Could you check a few things on this model? Use its own coordinates, in mm. A direction names the side the tool comes from. Coordinates: 2 decimals unless noted, no trailing zeros. Write each loop counter-clockwise with the first axis right and the second up, starting at its lowest first coordinate (ties: lowest second). Pieces come first, ordered by that corner, then holes. Notation, with made-up numbers: M 63.5,40 L 84.5,40 A30 cw 84.5,70 Z; hole C 48.25,49.5 d5. An arc over 180 degrees is marked long. Write item = value, one per line.
```python
from build123d import *

# Parameters (mm, degrees)
F1_DEPTH = 45
F2_T     = -2.5
F3_R     = 18
F4_DEPTH = 25
F5_R     = 20
F5_R_2   = 18
F6_DEPTH = 6


with BuildPart() as f1:
    # F0 (on Front) → F1 (new body)
    with BuildSketch(Plane.XZ):
        with BuildLine():
            Line((-26.5, -37.5), (26.5, -37.5))
            Line((26.5, -37.5), (26.5, 22.5))
            ThreePointArc((26.5, 22.5), (22.106602, 33.106602), (11.5, 37.5))
            Line((11.5, 37.5), (-11.5, 37.5))
            ThreePointArc((-11.5, 37.5), (-22.106602, 33.106602), (-26.5, 22.5))
            Line((-26.5, 22.5), (-26.5, -37.5))
        make_face()
    extrude(amount=F1_DEPTH)

    # F2
    f2_openings = [f1.faces().sort_by_distance(p)[0] for p in [
        (0, -45, -0.850304),
    ]]
    offset(amount=F2_T, openings=f2_openings)

    # F3 (on face) → F4 (cut)
    with BuildSketch(Plane(origin=(0, 0, 0), x_dir=(-1, 0, 0), z_dir=(0, 1, 0))):
        with Locations((0, 13)):
            Circle(F3_R)
    extrude(amount=-F4_DEPTH, mode=Mode.SUBTRACT)

    # F5 (on face) → F6 (join)
    with BuildSketch(Plane(origin=(0, 0, 0), x_dir=(-1, 0, 0), z_dir=(0, 1, 0))):
        with Locations((0, 13)):
            Circle(F5_R)
        with Locations((0, 13)):
            Circle(F5_R_2, mode=Mode.SUBTRACT)
    extrude(amount=F6_DEPTH)


solid = f1.part
```
Item 1: For faces 1 (the face through (-26.5, -22, -7)), 2 (the face through (-20.241, -23.452, 31.435)), which set-ups out of +Z, -Z, +X, -X, +Y, -Y let a thin tool reach every point of the face, with its end or its side?
Numbers:
face_1 = +Z, -Z, -X, +Y, -Y
face_2 = -Y
Item 2: Imagine slicing it at B-B (z = 13). Write out the boundary of the cut face in (x, y), and give its area (3 significant figures).
Numbers:
outline = M -26.5,-45 L -24,-45 L -24,-2.5 L -18,-2.5 L -18,6 L -20,6 L -20,0 L -26.5,0 Z; M 18,-2.5 L 24,-2.5 L 24,-45 L 26.5,-45 L 26.5,0 L 20,0 L 20,6 L 18,6 Z
area = 279 mm²
Item 3: If we mould it in two halves opening along Z, with no side actions, what happens to faces 3 (the face through (22.22, -22.18, 32.99)), 4 (the face through (-9.229, 2.958, -4.743)), 5 (the face through (-24, -23, -6))? For each: pulls with the +Z half, pulls with the -Z half, needs draft (parallel to the pull), parting line crosses it, or undercut.
Numbers:
face_3 = pulls with the +Z half
face_4 = parting line crosses it
face_5 = undercut
Item 4: Imagine slicing it at C-C (y = -24.5). Write out the boundary of the cut face in (x, z), and give its area (3 significant figures).
Numbers:
outline = M -26.5,-37.5 L 26.5,-37.5 L 26.5,22.5 A15 ccw 11.5,37.5 L -11.5,37.5 A15 ccw -26.5,22.5 Z; hole M -24,-35 L 24,-35 L 24,22.5 A12.5 ccw 11.5,35 L -11.5,35 A12.5 ccw -24,22.5 Z
area = 585 mm²
Item 5: I'm going to push flat-ended pins straight in: P1, Ø2, axis at x = 4, z = -26.5, coming from the -Y side; P2, Ø3, axis at x = 11.5, z = -10, coming from the +Y side. Where does each tip first touch, or does it pass through?
Numbers:
P1 = -2.5
P2 = 0
Item 6: Imagine slicing it at A-A (x = 0). Write out the boundary of the cut face in (y, z).
Numbers:
outline = M -45,-37.5 L 0,-37.5 L 0,-7 L 6,-7 L 6,-5 L -2.5,-5 L -2.5,-35 L -45,-35 Z; M -45,35 L -2.5,35 L -2.5,31 L 6,31 L 6,33 L 0,33 L 0,37.5 L -45,37.5 Z
Item 7: If I drill on line 1 along Z through (x, y) = (-10, -23.5); line 2 along X through (y, z) = (-32.5, -20); line 3 along Z through (x, y) = (0, -1), over which ranges is the centre line in solid material (lowest first)?
Numbers:
line_1 = -37.5 to -35, 35 to 37.5
line_2 = -26.5 to -24, 24 to 26.5
line_3 = -37.5 to -5, 31 to 37.5
Item 8: Imagine slicing it at D-D (z = -15.5). Write out the boundary of the cut face in (x, y).
Numbers:
outline = M -26.5,-45 L -24,-45 L -24,-2.5 L 24,-2.5 L 24,-45 L 26.5,-45 L 26.5,0 L -26.5,0 Z
